Source: three-view drawing plus pictorial views. Frame: mm from the lowest corner of the part. A direction names the side the tool comes from. Round coordinates to 2 decimals unless told otherwise and drop trailing zeros. Loops run counter-clockwise (first coordinate to the right, second up) from the corner with the lowest first, then second, coordinate; pieces in that order, holes last. Notation, with made-up numbers: M 21,-2.75 L 54,-2.75 A32 ccw 54,28.25 Z; hole C 42.25,-8 d8. An arc over 180 degrees is marked long. Write each question's results on one line, items separated by ' | '.
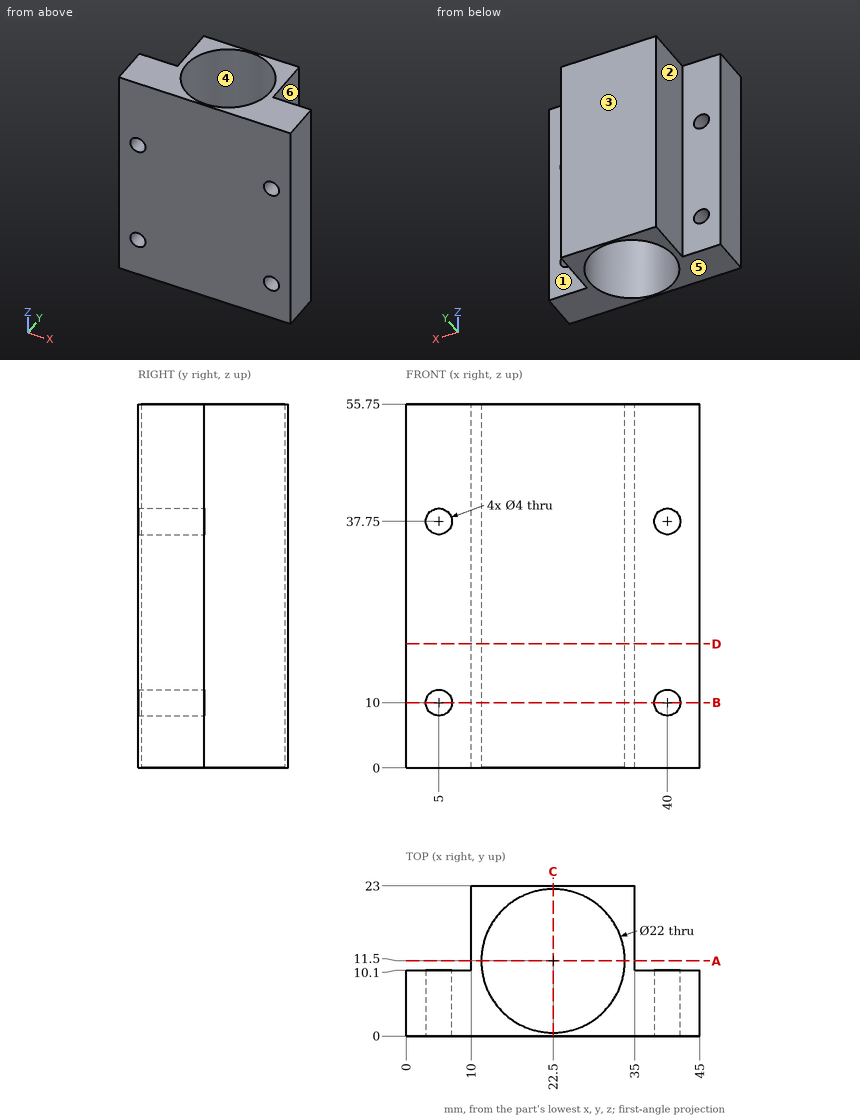
1. Section D-D (z = 19). Output: boundary loops of the cut face in (x, y).
Answer key:
outline: M 0,0 L 45,0 L 45,10.1 L 35,10.1 L 35,23 L 10,23 L 10,10.1 L 0,10.1 Z; hole C 22.5,11.5 d22
2. Section B-B (z = 10). Output: boundary loops of the cut face in (x, y), then the cut area to 3 significant figures.
Answer key:
outline: M 0,0 L 3,0 L 3,10.1 L 0,10.1 Z; M 7,0 L 38,0 L 38,10.1 L 35,10.1 L 35,23 L 10,23 L 10,10.1 L 7,10.1 Z; M 42,0 L 45,0 L 45,10.1 L 42,10.1 Z; hole C 22.5,11.5 d22 | area: 316 mm²
3. Section C-C (x = 22.5). Output: boundary loops of the cut face in (y, z).
Answer key:
outline: M 0,0 L 0.5,0 L 0.5,55.75 L 0,55.75 Z; M 22.5,0 L 23,0 L 23,55.75 L 22.5,55.75 Z
4. Ray query, probe 1 along Z at (x, y) = (5, 2.5); probe 2 along Z at (x, y) = (4, 4); probe 3 along Y at (x, z) = (23, 4). Return the intervals inside material, ascending.
Answer key:
probe 1: z = 0 to 8, 12 to 35.75, 39.75 to 55.75 | probe 2: z = 0 to 8.27, 11.73 to 36.02, 39.48 to 55.75 | probe 3: y = 0 to 0.51, 22.49 to 23
5. Pin query (flat end, axial travel): P1, Ø4, axis at y = 19.5, z = 32, coming from the +X side; P2, Ø11, axis at x = 3, z = 19.5, coming from the +Y side; P3, Ø3.5, axis at x = 5, z = 37.75, coming from the -Y side; P4, Ø4, axis at y = 18.5, z = 27.5, coming from the -X side. Return the tip coordinate at first contact, or that it passes through.
Answer key:
P1: stops at x = 35 | P2: stops at y = 10.1 | P3: passes through | P4: stops at x = 10
6. Section A-A (y = 11.5). Output: boundary loops of the cut face in (x, z).
Answer key:
outline: M 10,0 L 11.5,0 L 11.5,55.75 L 10,55.75 Z; M 33.5,0 L 35,0 L 35,55.75 L 33.5,55.75 Z
7. Draft query along X for the marked faces 4, 5 and 6. Return one class per face: pulls with the +X half, pulls with the -X half, needs draft (parallel to the pull), parting line crosses it, or undercut.
Answer key:
face 4: undercut | face 5: needs draft | face 6: pulls with the +X half
8. Access query for the marked faces 1, 2 and 3. Directions: +Z, -Z, +X, -X, +Y, -Y. A direction counts if a zero-diameter tool reaches every point of the face in a straight line with its end or side. Return the directions, or none.
Answer key:
face 1: +Z, -Z, +X, +Y | face 2: +Z, -Z, -X, +Y | face 3: +Z, -Z, +X, -X, +Y
